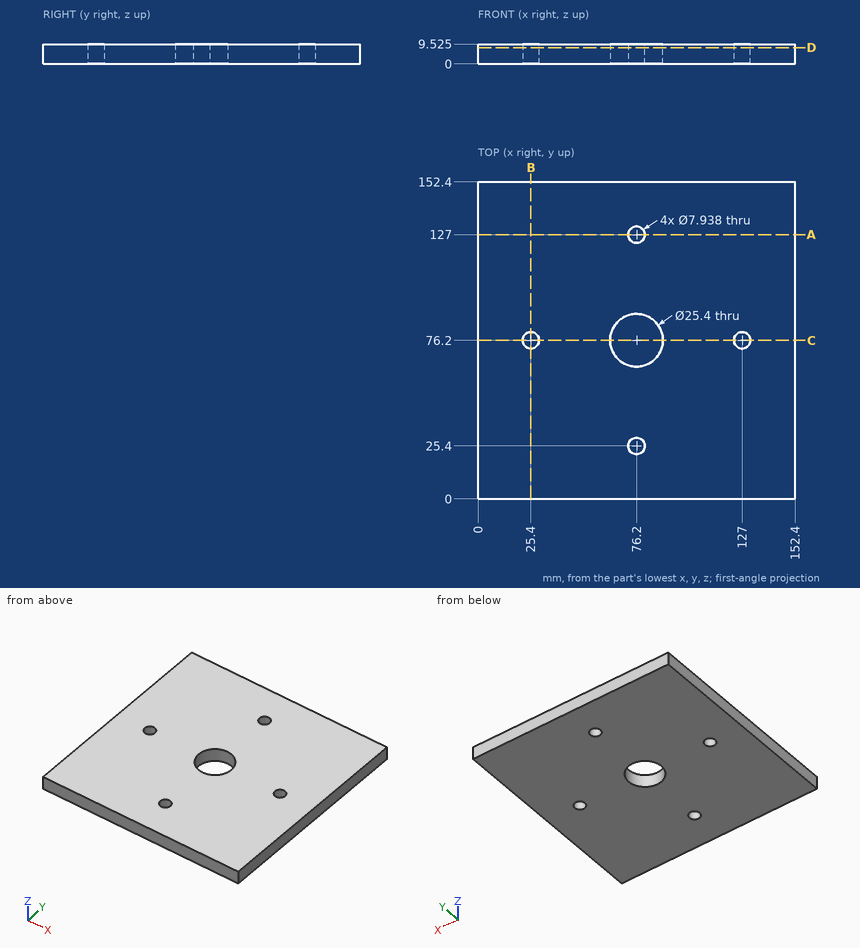
Design review of the part shown in the three views and the two pictorial views. Dimensions are in mm from the part's minimum x, y and z. Round coordinates to 2 decimals unless told otherwise and drop trailing zeros. Loops run counter-clockwise (first coordinate to the right, second up) from the corner with the lowest first, then second, coordinate; pieces in that order, holes last.
1) Consider section C-C on y = 76.2. State the section outline as (x, z) points (1 decimal).
Values follow:
outline: (0, 0) - (21.4, 0) - (21.4, 9.5) - (0, 9.5) - close; (29.4, 0) - (63.5, 0) - (63.5, 9.5) - (29.4, 9.5) - close; (88.9, 0) - (123, 0) - (123, 9.5) - (88.9, 9.5) - close; (131, 0) - (152.4, 0) - (152.4, 9.5) - (131, 9.5) - close
2) Clearance check with a flat-ended pin moving along its axis: P1, Ø20.5, axis at x = 76.2, y = 76.2, coming from the +Z side. State where the tip first meets the part, or that it passes through.
Values follow:
P1: passes through
3) Consider section D-D on z = 7.75. State the section outline as (x, y) points, then the cut area to 3 significant figures.
Values follow:
outline: (0, 0) - (152.4, 0) - (152.4, 152.4) - (0, 152.4) - close; hole circle Ø7.94 at (25.4, 76.2); hole circle Ø25.4 at (76.2, 76.2); hole circle Ø7.94 at (76.2, 25.4); hole circle Ø7.94 at (76.2, 127); hole circle Ø7.94 at (127, 76.2)
area: 22,500 mm2
4) Consider section A-A on y = 127. State the section outline as (x, z) points (1 decimal), then the cut area to 3 significant figures.
Values follow:
outline: (0, 0) - (72.2, 0) - (72.2, 9.5) - (0, 9.5) - close; (80.2, 0) - (152.4, 0) - (152.4, 9.5) - (80.2, 9.5) - close
area: 1,380 mm2
5) Wall thickness on line 1 along Y through (x, z) = (76.2, 7); line 2 along Y through (x, z) = (127, 6.5): over which ranges is each line inside the solid? List them lowest first.
Values follow:
line 1: y = 0 to 21.43, 29.37 to 63.5, 88.9 to 123.03, 130.97 to 152.4
line 2: y = 0 to 72.23, 80.17 to 152.4
